Answer from the drawing. Dimensions are ordinates in mm from the lowest x, y and z of the part. A direction names the side the tool comes from. Coordinates: 2 decimals unless noted, no trailing zeros. Loops run counter-clockwise (first coordinate to the right, second up) from the corner with the lowest first, then second, coordinate; pieces in that order, holes last. Notation, with made-up numbers: M -32,86.25 L 1,86.25 A18 cw 1,120.25 Z; hole C 22,66.25 d9. An arc over 180 degrees is marked long. Put each result on its own line as item: value.
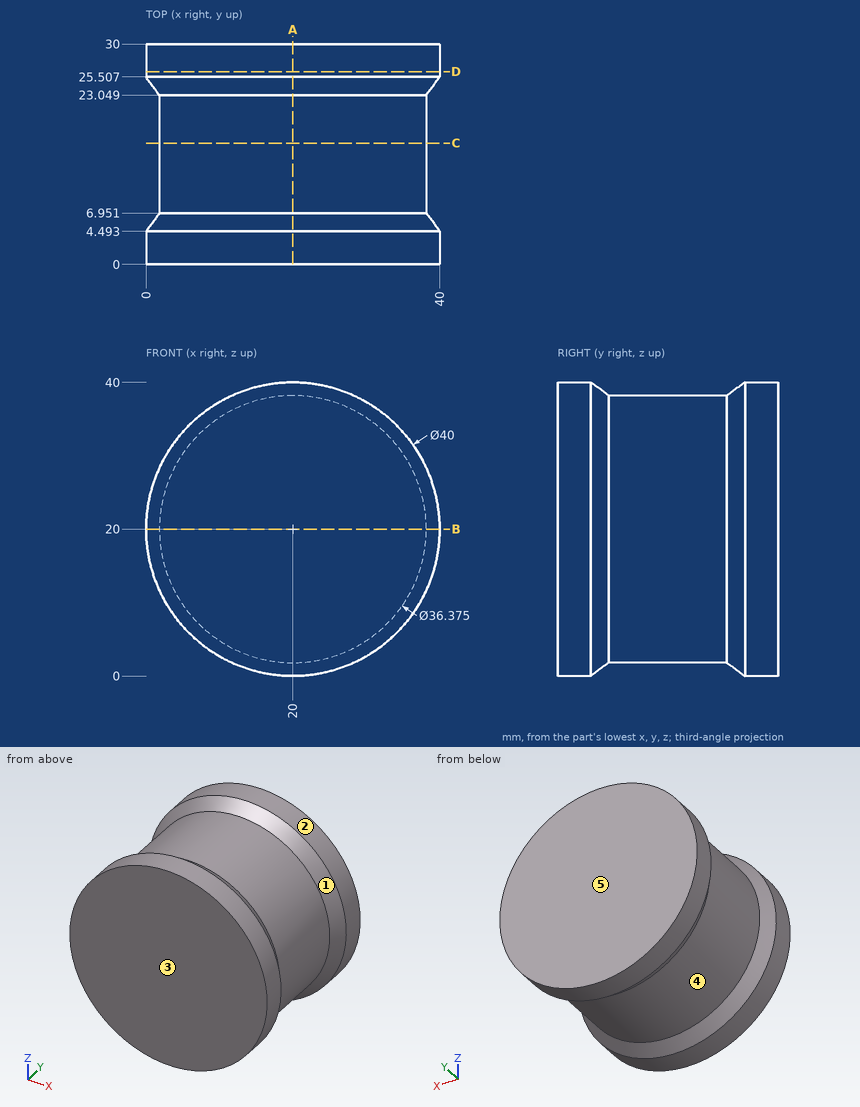
1) Determine the mould class of the marked faces 3, 4 and 5 for opening direction Y: released by +Y, released by -Y, zero draft, split by the parting line, or undercut.
Answer list:
face 3: released by -Y
face 4: undercut
face 5: released by +Y
2) Which of the six approach directions +Z, -Z, +X, -X, +Y, -Y give full straight-line access (tool end or side, diameter ignored) to the marked faces 1 and 2?
Answer list:
face 1: none
face 2: +Y, -Y
3) Straight lines are drawn through the part: line 1 (Y direction, x = 26.5, z = 38.5) (1 decimal); line 2 (X direction, y = 23.5, z = 30.5) (1 decimal); line 3 (X direction, y = 14.5, z = 21.5) (1 decimal). For each, find the intervals that lie inside material, in ascending order. Write a range as [from, to].
Answer list:
line 1: y = [0, 5], [25, 30]
line 2: x = [4.7, 35.3]
line 3: x = [1.9, 38.1]
4) Given pin 1 Ø6 at (y, z) = (19, 32.5) entering from -X; pin 2 Ø6 at (y, z) = (23, 35.5) entering from -X (1 decimal); pin 3 Ø1 at (x, z) = (33.5, 28) entering from -Y; pin 4 Ø1 at (x, y) = (34, 9.5) entering from -Z, each flat-ended and moving along its own axis, determine where each tip first touches the part or whether it passes through.
Answer list:
pin 1: stops at x = 4.49
pin 2: stops at x = 5.5
pin 3: stops at y = 0
pin 4: stops at z = 7.81
5) Find section B-B, the plane z = 20. Write down the section's boundary in (x, y).
Answer list:
outline: M 0,0 L 40,0 L 40,4.49 L 38.19,6.95 L 38.19,23.05 L 40,25.51 L 40,30 L 0,30 L 0,25.51 L 1.81,23.05 L 1.81,6.95 L 0,4.49 Z
6) Find section D-D, the plane y = 26.25. Write down the section's boundary in (x, z).
Answer list:
outline: C 20,20 d40
7) Find section A-A, the plane x = 20. Write down the section's boundary in (y, z).
Answer list:
outline: M 0,0 L 4.49,0 L 6.95,1.81 L 23.05,1.81 L 25.51,0 L 30,0 L 30,40 L 25.51,40 L 23.05,38.19 L 6.95,38.19 L 4.49,40 L 0,40 Z
8) Find section C-C, the plane y = 16.5. Write down the section's boundary in (x, z) (1 decimal).
Answer list:
outline: C 20,20 d36.4
